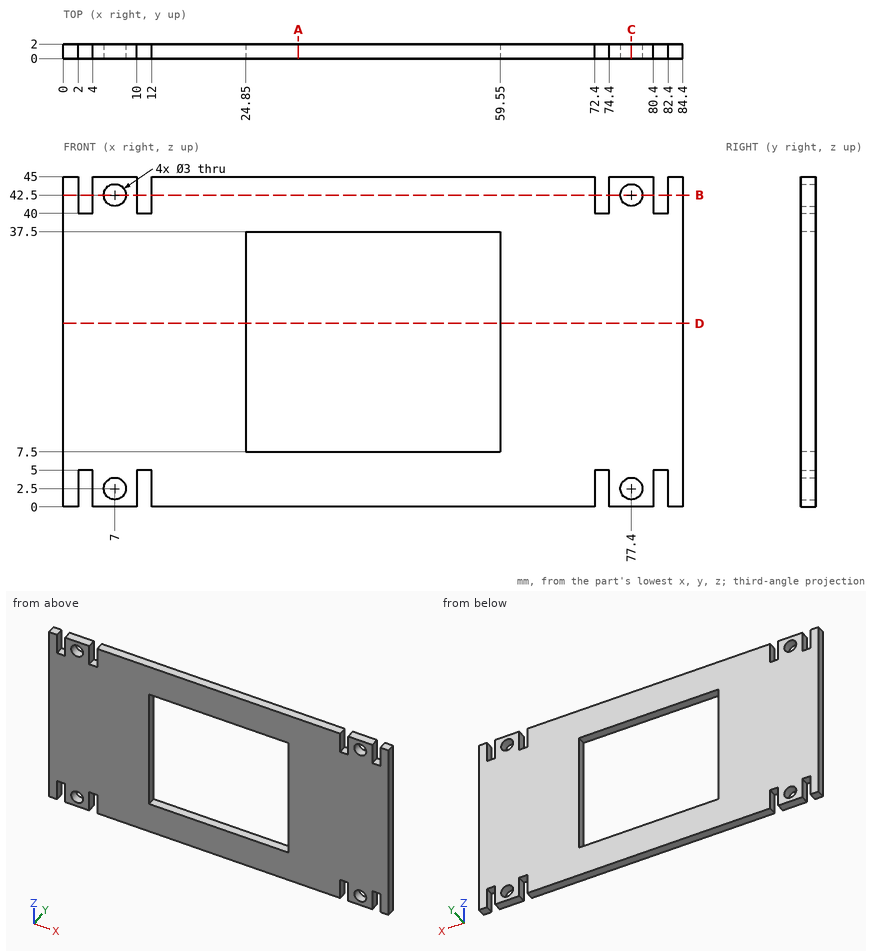
Source: three-view drawing plus pictorial views. Frame: mm from the lowest corner of the part. Round coordinates to 2 decimals unless told otherwise and drop trailing zeros. Loops run counter-clockwise (first coordinate to the right, second up) from the corner with the lowest first, then second, coordinate; pieces in that order, holes last.
1. Section query B-B on z = 42.5. Output: boundary loops of the cut face in (x, y), and give its area (3 significant figures).
2. Section query D-D on z = 25. Output: boundary loops of the cut face in (x, y), and give its area (3 significant figures).
3. Section query C-C on x = 77.4. Output: boundary loops of the cut face in (y, z), and give its area (3 significant figures).
4. Ray query, L1, parallel to Z at x = 37, y = 1; L2, parallel to X at y = 0.6, z = 16; L3, parallel to Z at x = 81.5, y = 1.1. Return the intervals inside material, ascending.
5. Section query A-A on x = 32. Output: boundary loops of the cut face in (y, z).
6. Contact query for a flat-ended pin moving along its axis: pin 1 (2.5 mm diameter, centred on x = 77.4, z = 2.5, fed in from -Y). Output: stop coordinate, or through.
Answers below:
1. outline: (0, 0) - (2, 0) - (2, 2) - (0, 2) - close; (4, 0) - (5.5, 0) - (5.5, 2) - (4, 2) - close; (8.5, 0) - (10, 0) - (10, 2) - (8.5, 2) - close; (12, 0) - (72.4, 0) - (72.4, 2) - (12, 2) - close; (74.4, 0) - (75.9, 0) - (75.9, 2) - (74.4, 2) - close; (78.9, 0) - (80.4, 0) - (80.4, 2) - (78.9, 2) - close; (82.4, 0) - (84.4, 0) - (84.4, 2) - (82.4, 2) - close
1. area: 141 mm2
2. outline: (0, 0) - (24.85, 0) - (24.85, 2) - (0, 2) - close; (59.55, 0) - (84.4, 0) - (84.4, 2) - (59.55, 2) - close
2. area: 99.4 mm2
3. outline: (0, 0) - (2, 0) - (2, 1) - (0, 1) - close; (0, 4) - (2, 4) - (2, 41) - (0, 41) - close; (0, 44) - (2, 44) - (2, 45) - (0, 45) - close
3. area: 78.0 mm2
4. L1: z = 0 to 7.5, 37.5 to 45
4. L2: x = 0 to 24.85, 59.55 to 84.4
4. L3: z = 5 to 40
5. outline: (0, 0) - (2, 0) - (2, 7.5) - (0, 7.5) - close; (0, 37.5) - (2, 37.5) - (2, 45) - (0, 45) - close
6. pin 1: passes through
